Part model, mm, in its own coordinate system. A direction names the side the tool comes from. Coordinates: 2 decimals unless noted, no trailing zeros. Order: outer loops, then holes, each group sorted by start corner. A loop starts at its lowest first (then second) coordinate and runs counter-clockwise, first axis right, second up.
from build123d import *

# Parameters (mm, degrees)
SKETCH1_R           = 1.6
SKETCH1_R_2         = 21.732875
SKETCH1_R_3         = 19.192875
BOSS_EXTRUDE1_DEPTH = 11.05
BOSS_EXTRUDE2_START = 11.05
SKETCH1_3_R         = 21.732875
SKETCH1_3_R_2       = 19.192875
BOSS_EXTRUDE2_DEPTH = 7.62
CUT_EXTRUDE1_DEPTH  = 42.937776077
FILLET2_R           = 0.79375
FILLET4_R           = 2.54
FILLET5_R           = 2.54
FILLET6_R           = 2.54
FILLET7_R           = 2.54
BOSS_EXTRUDE3_DEPTH = 11.05


with BuildPart() as part:
    # Sketch1 → Boss-Extrude1 (new body)
    # profile 1 of 6: a face of its own
    with BuildSketch(Plane(origin=(0, 0, 0), x_dir=(1, 0, 0), z_dir=(0, 1, 0))):
        with BuildLine():
            Line((-8.562572408, 19.9749896), (-25.4, 19.9749896))
            ThreePointArc((-25.4, 19.9749896), (-30.6249948, 14.7499948), (-25.4, 9.525))
            Line((-25.4, 9.525), (-19.534385856, 9.525))
            ThreePointArc((-19.534385856, 9.525), (-14.98867361, 15.737138215), (-8.562572408, 19.9749896))
        make_face()
        with Locations(Location((-25.4, 14.7499948, 0), (0, 0, 270))):
            Circle(SKETCH1_R, mode=Mode.SUBTRACT)
    # profile 2 of 6: a face of its own
    with BuildSketch(Plane(origin=(0, 0, 0), x_dir=(1, 0, 0), z_dir=(0, 1, 0))):
        Circle(SKETCH1_R_2)
        Circle(SKETCH1_R_3, mode=Mode.SUBTRACT)
    # profile 3 of 6: a face of its own
    with BuildSketch(Plane(origin=(0, 0, 0), x_dir=(1, 0, 0), z_dir=(0, 1, 0))):
        with BuildLine():
            Line((25.4, 19.9749896), (8.562572408, 19.9749896))
            ThreePointArc((8.562572408, 19.9749896), (14.98867361, 15.737138215), (19.534385856, 9.525))
            Line((19.534385856, 9.525), (25.4, 9.525))
            ThreePointArc((25.4, 9.525), (30.6249948, 14.7499948), (25.4, 19.9749896))
        make_face()
        with Locations(Location((25.4, 14.7499948, 0), (0, 0, 270))):
            Circle(SKETCH1_R, mode=Mode.SUBTRACT)
    # profile 4 of 6: a face of its own
    with BuildSketch(Plane(origin=(0, 0, 0), x_dir=(1, 0, 0), z_dir=(0, 1, 0))):
        with BuildLine():
            Line((25.4, -9.525), (19.534385856, -9.525))
            ThreePointArc((19.534385856, -9.525), (14.98867361, -15.737138215), (8.562572408, -19.9749896))
            Line((8.562572408, -19.9749896), (25.4, -19.9749896))
            ThreePointArc((25.4, -19.9749896), (30.6249948, -14.7499948), (25.4, -9.525))
        make_face()
        with Locations(Location((25.4, -14.7499948, 0), (0, 0, 270))):
            Circle(SKETCH1_R, mode=Mode.SUBTRACT)
    # profile 5 of 6: a face of its own
    with BuildSketch(Plane(origin=(0, 0, 0), x_dir=(1, 0, 0), z_dir=(0, 1, 0))):
        with BuildLine():
            ThreePointArc((-8.562572408, -19.9749896), (-14.98867361, -15.737138215), (-19.534385856, -9.525))
            Line((-19.534385856, -9.525), (-25.4, -9.525))
            ThreePointArc((-25.4, -9.525), (-30.6249948, -14.7499948), (-25.4, -19.9749896))
            Line((-25.4, -19.9749896), (-8.562572408, -19.9749896))
        make_face()
        with Locations(Location((-25.4, -14.7499948, 0), (0, 0, 270))):
            Circle(SKETCH1_R, mode=Mode.SUBTRACT)
    # profile 6 of 6: a face of its own
    with BuildSketch(Plane(origin=(0, 0, 0), x_dir=(1, 0, 0), z_dir=(0, 1, 0))):
        Circle(SKETCH1_R_3)
    extrude(amount=BOSS_EXTRUDE1_DEPTH)

    # Sketch1<3> → Boss-Extrude2 (add)
    with BuildSketch(Plane(origin=(0, 0, 0), x_dir=(1, 0, 0), z_dir=(0, 1, 0)).offset(BOSS_EXTRUDE2_START)):
        with Locations(Location((0, 0, 0), (0, 0, 113.203103919))):
            Circle(SKETCH1_3_R)
        with Locations(Location((0, 0, 0), (0, 0, 90))):
            Circle(SKETCH1_3_R_2, mode=Mode.SUBTRACT)
    extrude(amount=BOSS_EXTRUDE2_DEPTH)

    # Sketch2 → Cut-Extrude1 (cut, through all)
    with BuildSketch(Plane(origin=(0, 18.67, 0), x_dir=(1, 0, 0), z_dir=(0, 1, 0))):
        with BuildLine():
            Line((-19.534385856, 9.525), (-16.6625576, 9.525))
            ThreePointArc((-16.6625576, 9.525), (-19.192875, 0), (-16.6625576, -9.525))
            Line((-16.6625576, -9.525), (-19.534385856, -9.525))
            ThreePointArc((-19.534385856, -9.525), (-21.732875, 0), (-19.534385856, 9.525))
        make_face()
        with BuildLine():
            Line((19.534385856, 9.525), (16.6625576, 9.525))
            ThreePointArc((16.6625576, 9.525), (19.192875, 0), (16.6625576, -9.525))
            Line((16.6625576, -9.525), (19.534385856, -9.525))
            ThreePointArc((19.534385856, -9.525), (21.732875, 0), (19.534385856, 9.525))
        make_face()
        with BuildLine():
            Line((-8.562572408, 19.9749896), (-7.561833485, 17.640440049))
            ThreePointArc((-7.561833485, 17.640440049), (0, 19.192875), (7.561833485, 17.640440049))
            Line((7.561833485, 17.640440049), (8.562572408, 19.9749896))
            ThreePointArc((8.562572408, 19.9749896), (0, 21.732875), (-8.562572408, 19.9749896))
        make_face()
        with BuildLine():
            Line((-8.562572408, -19.9749896), (-7.561833485, -17.640440049))
            ThreePointArc((-7.561833485, -17.640440049), (0, -19.192875), (7.561833485, -17.640440049))
            Line((7.561833485, -17.640440049), (8.562572408, -19.9749896))
            ThreePointArc((8.562572408, -19.9749896), (0, -21.732875), (-8.562572408, -19.9749896))
        make_face()
    extrude(amount=-CUT_EXTRUDE1_DEPTH, mode=Mode.SUBTRACT)

    # Fillet2
    fillet2_edges = [part.edges().sort_by_distance(p)[0] for p in [
        (16.6625576, 14.86, 9.525),
        (19.534385856, 14.86, -9.525),
        (19.534385856, 14.86, 9.525),
        (16.6625576, 14.86, -9.525),
        (7.561833485, 14.86, -17.640440049),
        (-8.562572408, 14.86, -19.9749896),
        (8.562572408, 14.86, -19.9749896),
        (-7.561833485, 14.86, -17.640440049),
        (-16.6625576, 14.86, -9.525),
        (-19.534385856, 14.86, 9.525),
        (-19.534385856, 14.86, -9.525),
        (-16.6625576, 14.86, 9.525),
        (-7.561833485, 14.86, 17.640440049),
        (8.562572408, 14.86, 19.9749896),
        (-8.562572408, 14.86, 19.9749896),
        (7.561833485, 14.86, 17.640440049),
    ]]
    fillet(fillet2_edges, radius=FILLET2_R)

    # Fillet4
    # the kernel refuses this fillet: 2.54 mm, written as the material it adds along each edge
    with BuildSketch(Plane(origin=(16.6625576, 11.05, 9.525), x_dir=(1, 0, 0), z_dir=(0, -1, 0))) as fillet4_piece_1:
        with BuildLine():
            CenterArc((3.917229347, -2.54), FILLET4_R, 90, 108.747762366)
            ThreePointArc((1.511994934, -3.356362308), (0.836652457, -1.641847194), (0, 0))
            Line((0, 0), (3.917229347, 0))
        make_face()
    extrude(amount=11.05)

    # Fillet5
    # the kernel refuses this fillet: 2.54 mm, written as the material it adds along each edge
    with BuildSketch(Plane(origin=(16.6625576, 11.05, -9.525), x_dir=(0.41073329589504654, 0, 0.9117555372155368), z_dir=(0, -1, 0))) as fillet5_piece_1:
        with BuildLine():
            CenterArc((3.924795585, -2.528292976), FILLET5_R, 95.503145264, 108.747762366)
            Line((1.60893652, -3.571555547), (0, 0))
            ThreePointArc((0, 0), (1.840604291, -0.088461201), (3.681208582, 0))
        make_face()
    extrude(amount=11.05)

    # Fillet6
    # the kernel refuses this fillet: 2.54 mm, written as the material it adds along each edge
    with BuildSketch(Plane(origin=(-16.6625576, 11.05, -9.525), x_dir=(-1, 0, 0), z_dir=(0, -1, 0))) as fillet6_piece_1:
        with BuildLine():
            CenterArc((3.917229347, -2.54), FILLET6_R, 90, 108.747762366)
            ThreePointArc((1.511994934, -3.356362308), (0.836652457, -1.641847194), (0, 0))
            Line((0, 0), (3.917229347, 0))
        make_face()
    extrude(amount=11.05)

    # Fillet7
    # the kernel refuses this fillet: 2.54 mm, written as the material it adds along each edge
    with BuildSketch(Plane(origin=(-16.6625576, 11.05, 9.525), x_dir=(-0.41073329589504604, 0, -0.9117555372155371), z_dir=(0, -1, 0))) as fillet7_piece_1:
        with BuildLine():
            CenterArc((3.924795585, -2.528292976), FILLET7_R, 95.503145264, 108.747762366)
            Line((1.60893652, -3.571555547), (0, 0))
            ThreePointArc((0, 0), (1.840604291, -0.088461201), (3.681208582, 0))
        make_face()
    extrude(amount=11.05)

    # Sketch3 → Boss-Extrude3 (add)
    with BuildSketch(Plane(origin=(0, 11.05, 0), x_dir=(1, 0, 0), z_dir=(0, 1, 0))):
        with BuildLine():
            ThreePointArc((9.7e-08, 19.192875), (3.859772707, 18.800760767), (7.561833485, 17.640440049))
            Line((7.561833485, 17.640440049), (8.562572408, 19.9749896))
            ThreePointArc((8.562572408, 19.9749896), (4.299108953, 19.388809795), (9.7e-08, 19.192875))
        make_face()
        with BuildLine():
            ThreePointArc((-7.561833485, 17.640440049), (-3.859772612, 18.800760786), (9.7e-08, 19.192875))
            ThreePointArc((9.7e-08, 19.192875), (-4.299108856, 19.388809786), (-8.562572408, 19.9749896))
            Line((-8.562572408, 19.9749896), (-7.561833485, 17.640440049))
        make_face()
        with BuildLine():
            ThreePointArc((7.561833485, -17.640440049), (3.859772707, -18.800760767), (9.7e-08, -19.192875))
            ThreePointArc((9.7e-08, -19.192875), (4.299108953, -19.388809795), (8.562572408, -19.9749896))
            Line((8.562572408, -19.9749896), (7.561833485, -17.640440049))
        make_face()
        with BuildLine():
            Line((-7.561833485, -17.640440049), (-8.562572408, -19.9749896))
            ThreePointArc((-8.562572408, -19.9749896), (-4.299108856, -19.388809786), (9.7e-08, -19.192875))
            ThreePointArc((9.7e-08, -19.192875), (-3.859772612, -18.800760786), (-7.561833485, -17.640440049))
        make_face()
    extrude(amount=-BOSS_EXTRUDE3_DEPTH)


solid = part.part
Q1. Cut at B-B on y = 15.5. Count the separate pieces of the cut face and the enclosed holes in it, and give its area (3 significant figures).
Results list:
separate pieces: 4
enclosed holes: 0
area: 139 mm2
Q2. Mould opens along Z. For faces 1 (the face through (-12.95, 14.807, 14.166)), 2 (the face through (14.87, 14.81, -15.85)), 3 (the face through (-17, 5, 19.975)) say: pulls with the +Z half, pulls with the -Z half, needs draft (parallel to the pull), parting line crosses it, or undercut.
Results list:
face 1: undercut
face 2: pulls with the -Z half
face 3: pulls with the +Z half
Q3. Cut at C-C on z = 14. Write the cut outline in (x, y), and give its area (3 significant figures).
Results list:
outline: (-30.57, 0) - (-26.81, 0) - (-26.81, 11.05) - (-30.57, 11.05) - close; (-23.99, 0) - (23.99, 0) - (23.99, 11.05) - (16.62, 11.05) - (16.62, 18.67) - (13.13, 18.67) - (13.13, 11.05) - (-13.13, 11.05) - (-13.13, 18.67) - (-16.62, 18.67) - (-16.62, 11.05) - (-23.99, 11.05) - close; (26.81, 0) - (30.57, 0) - (30.57, 11.05) - (26.81, 11.05) - close
area: 666 mm2
Q4. Cut at D-D on y = 9.25. Write the cut outline in (x, z) (3 decimals).
Results list:
outline: (-25.4, -19.975) - (-8.563, -19.975) arc R47.262 cw to (8.563, -19.975) - (25.4, -19.975) arc R5.225 ccw to (25.4, -9.525) - (20.58, -9.525) arc R2.54 cw to (18.175, -6.169) arc R19.193 ccw to (18.175, 6.169) arc R2.54 cw to (20.58, 9.525) - (25.4, 9.525) arc R5.225 ccw to (25.4, 19.975) - (8.563, 19.975) arc R47.262 cw to (-8.563, 19.975) - (-25.4, 19.975) arc R5.225 ccw to (-25.4, 9.525) - (-20.58, 9.525) arc R2.54 cw to (-18.175, 6.169) arc R19.193 ccw to (-18.175, -6.169) arc R2.54 cw to (-20.58, -9.525) - (-25.4, -9.525) arc R5.225 ccw to start; hole circle Ø3.2 at (-25.4, -14.75); hole circle Ø3.2 at (-25.4, 14.75); hole circle Ø3.2 at (25.4, -14.75); hole circle Ø3.2 at (25.4, 14.75)
Q5. Pin check, flat tips, straight feed: pin 1 Ø1.2 at (x, y) = (-17.5, 16) entering from -Z; pin 2 Ø6 at (y, z) = (11.5, -7.5) entering from +X; pin 3 Ø3 at (x, z) = (-25.4, -14.75) entering from -Y; pin 4 Ø20 at (x, z) = (13.5, 8) entering from +Y. Stop position of each tip, or through.
Results list:
pin 1: stops at z = -13.66
pin 2: stops at x = 28.39
pin 3: passes through
pin 4: stops at y = 18.67
Q6. Which spindle directions (+Z, -Z, +X, -X, +Y, -Y) get a long thin tool onto all of the face, cutting with end or side? Do faces 4 (the face through (23, 6, 9.525)), 5 (the face through (-23, 6, -9.525)), 6 (the face through (12.8, 14.8, 14.3)), 7 (the face through (-14.87, 14.81, 15.85)), 8 (the face through (18.9, 14.81, -9.91)). Say none if no direction does.
Results list:
face 4: +X, +Y, -Y
face 5: -X, +Y, -Y
face 6: +Y
face 7: +Z, -X, +Y
face 8: +X, +Y
Q7. Cut at A-A on x = -22.5. Write the cut outline in (y, z) (3 decimals), and give its area (3 significant figures).
Results list:
outline: (0, -19.975) - (11.05, -19.975) - (11.05, -9.525) - (0, -9.525) - close; (0, 9.525) - (11.05, 9.525) - (11.05, 19.975) - (0, 19.975) - close
area: 231 mm2
Q8. Wall check: line 1 along Z through (x, y) = (22, 1.25) (3 decimals); line 2 along X through (y, z) = (7, 14); line 3 along X through (y, z) = (9, 15). Give the ranges that are in metal, low to high.
Results list:
line 1: z = -19.975 to -9.525, 9.525 to 19.975
line 2: x = -30.57 to -26.81, -23.99 to 23.99, 26.81 to 30.57
line 3: x = -30.62 to -26.98, -23.82 to 23.82, 26.98 to 30.62
